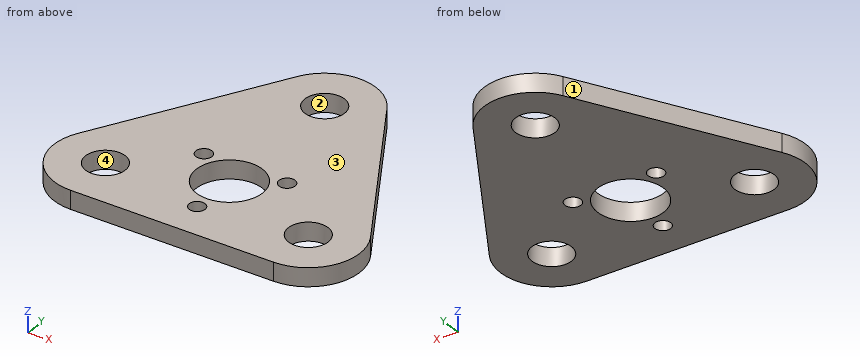
from build123d import *

# Parameters (mm, degrees)
SKETCH1_R           = 7.5
SKETCH1_R_2         = 12.5
SKETCH1_R_3         = 3
SKETCH1_R_4         = 3.042653236
BOSS_EXTRUDE1_DEPTH = 7


with BuildPart() as part:
    # Sketch1 → Boss-Extrude1 (new body)
    with BuildSketch(Plane.XY):
        with BuildLine():
            Line((-16.819672131, 55.195439587), (-54.819672131, -10.622491101))
            ThreePointArc((-54.819672131, -10.622491101), (-54.819672131, -30.044175566), (-38, -39.755017799))
            Line((-38, -39.755017799), (38, -39.755017799))
            ThreePointArc((38, -39.755017799), (54.819672131, -30.044175566), (54.819672131, -10.622491101))
            Line((54.819672131, -10.622491101), (16.819672131, 55.195439587))
            ThreePointArc((16.819672131, 55.195439587), (0, 64.906281819), (-16.819672131, 55.195439587))
        make_face()
        with Locations((0, 45.484597354)):
            Circle(SKETCH1_R, mode=Mode.SUBTRACT)
        with Locations((38, -20.333333333)):
            Circle(SKETCH1_R, mode=Mode.SUBTRACT)
        with Locations((-38, -20.333333333)):
            Circle(SKETCH1_R, mode=Mode.SUBTRACT)
        with Locations((0, -7.755017799)):
            Circle(SKETCH1_R_2, mode=Mode.SUBTRACT)
        with Locations((0, -25.755017799)):
            Circle(SKETCH1_R_3, mode=Mode.SUBTRACT)
        with Locations((-15.588457268, 1.244982201)):
            Circle(SKETCH1_R_4, mode=Mode.SUBTRACT)
        with Locations(Location((15.588457268, 1.244982201, 0), (0, 0, 180))):
            Circle(SKETCH1_R_4, mode=Mode.SUBTRACT)
    extrude(amount=BOSS_EXTRUDE1_DEPTH)


solid = part.part
Work out the finished part from the listing and answer in its coordinate system (mm). Face numbers are marked on the shaded views. Give positions to 0.01 mm unless a question says otherwise; leave off trailing zeros. Write each loop counter-clockwise with the first axis right and the second up, starting at its lowest first coordinate (ties: lowest second). Pieces come first, ordered by that corner, then holes. Notation, with made-up numbers: (25, -5.5) - (78, -5.5) arc R19 cw to (78, 7.5) - close; hole circle Ø11 at (89.5, 28). An arc over 180 degrees is marked (long way). One line per item, written item: value. Start each with the question number.
1. Find section A-A (y = -5.5). Write down the section's boundary in (x, z).
2. Consider probe 1 along X at (y, z) = (-14.5, 1); probe 2 along Y at (x, z) = (-6, 3); probe 3 along Y at (x, z) = (-1, 4.5). Determine where each line is inside the solid, lowest interval first.
3. Find section B-B (x = 0). Write down the section's boundary in (y, z).
4. Given pin 1 (4 mm diameter, centred on y = -21.5, z = 4, fed in from +X); pin 2 (22.5 mm diameter, centred on x = 0, y = -7.76, fed in from +Z); pin 3 (2 mm diameter, centred on y = -25.5, z = 4.5, fed in from -X); pin 4 (4 mm diameter, centred on y = 6, z = 4.5, fed in from +X), each flat-ended and moving along its own axis, determine where each tip first touches the part or whether it passes through.
5. Find section C-C (z = 2.5). Write down the section's boundary in (x, y).
6. Find section D-D (x = -36). Write down the section's boundary in (y, z).
7. For a pull along Y with two mould halves and no side action, classify the marked faces 1, 2, 3 and 4 as +Y half, -Y half, draft (parallel to the pull), parting line (faces both ways), or undercut.
Geometry results:
1. outline: (-51.86, 0) - (-12.29, 0) - (-12.29, 7) - (-51.86, 7) - close; (12.29, 0) - (51.86, 0) - (51.86, 7) - (12.29, 7) - close
2. probe 1: -56.52 to -42.71, -33.29 to -10.52, 10.52 to 33.29, 42.71 to 56.52
2. probe 2: -39.76 to -18.72, 3.21 to 40.98, 49.98 to 63.96
2. probe 3: -39.76 to -28.58, -22.93 to -20.21, 4.7 to 38.05, 52.92 to 64.88
3. outline: (-39.76, 0) - (-28.76, 0) - (-28.76, 7) - (-39.76, 7) - close; (-22.76, 0) - (-20.26, 0) - (-20.26, 7) - (-22.76, 7) - close; (4.74, 0) - (37.98, 0) - (37.98, 7) - (4.74, 7) - close; (52.98, 0) - (64.91, 0) - (64.91, 7) - (52.98, 7) - close
4. pin 1: x = 57.42
4. pin 2: through
4. pin 3: x = -56.97
4. pin 4: x = 46.38
5. outline: (-54.82, -10.62) arc R19.42 ccw to (-38, -39.76) - (38, -39.76) arc R19.42 ccw to (54.82, -10.62) - (16.82, 55.2) arc R19.42 ccw to (-16.82, 55.2) - close; hole circle Ø15 at (-38, -20.33); hole circle Ø6.09 at (-15.59, 1.24); hole circle Ø25 at (0, -7.76); hole circle Ø15 at (0, 45.48); hole circle Ø6 at (0, -25.76); hole circle Ø6.09 at (15.59, 1.24); hole circle Ø15 at (38, -20.33)
6. outline: (-39.76, 0) - (-27.56, 0) - (-27.56, 7) - (-39.76, 7) - close; (-13.1, 0) - (21.97, 0) - (21.97, 7) - (-13.1, 7) - close
7. face 1: +Y half
7. face 2: undercut
7. face 3: draft
7. face 4: undercut
